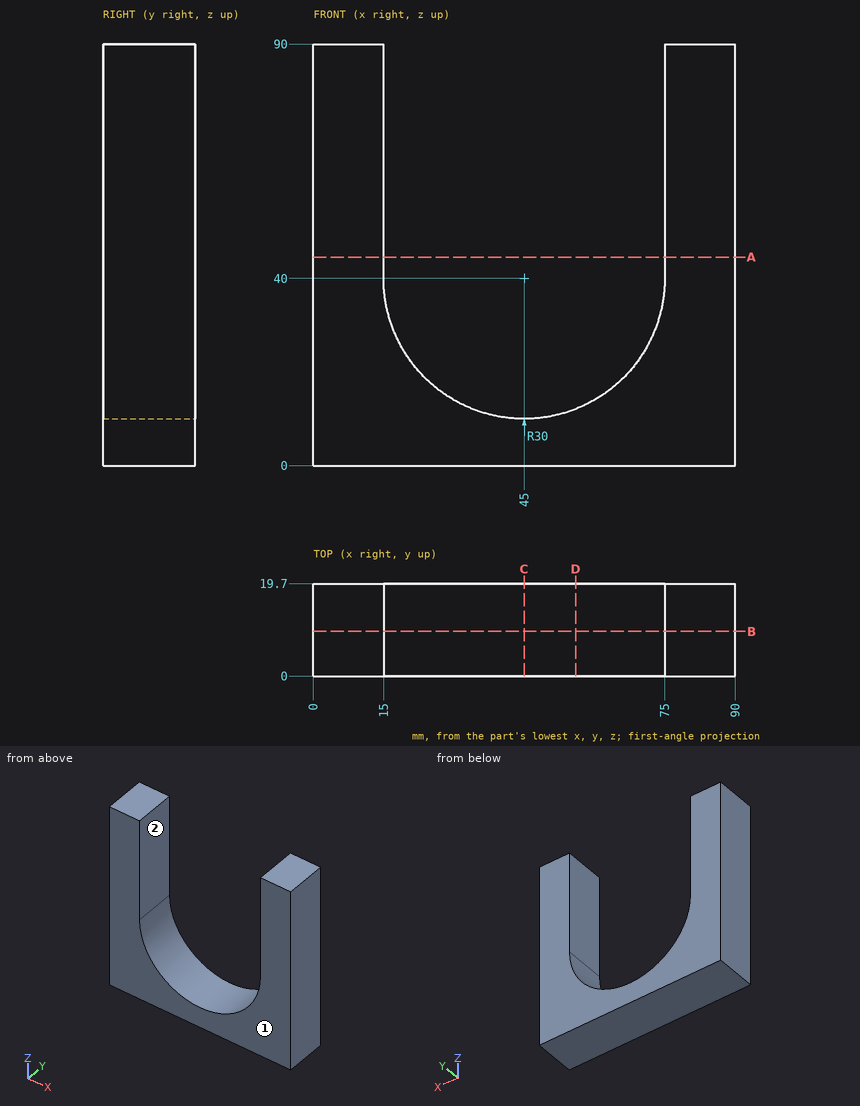
Geometry: see drawing. Coordinates: mm, zero at the bounding-box minimum. A direction names the side the tool comes from. Round coordinates to 2 decimals unless told otherwise and drop trailing zeros. Order: outer loops, then holes, each group sorted by start corner. A loop starts at its lowest first (then second) coordinate and runs counter-clockwise, first axis right, second up. Notation, with made-up numbers: (-16.5, 64.5) -> (21.5, 64.5) arc R25 ccw to (21.5, 100.5) -> close; hole circle Ø6 at (22, 1). An arc over 180 degrees is marked (long way). Use CSV: the item, a comma, the result in double quotes.
(1) Section C-C on x = 45. Return the cut outline in (y, z).
Report:
outline,"(0, 0) -> (19.7, 0) -> (19.7, 10) -> (0, 10) -> close"
(2) First-contact query: pin 1 Ø2 at (x, y) = (69, 16) entering from +Z; pin 2 Ø8 at (x, z) = (21.5, 73.5) entering from -Y; pin 3 Ø3 at (x, y) = (28, 8.5) entering from +Z. Flat tips, straight axial feed; report the tip coordinate or a pass-through.
Report:
pin 1,"z = 23.42"
pin 2,"through"
pin 3,"z = 16.38"
(3) Access query for the marked faces 1 and 2. Directions: +Z, -Z, +X, -X, +Y, -Y. A direction counts if a zero-diameter tool reaches every point of the face in a straight line with its end or side. Return the directions, or none.
Report:
face 1,"+Z, -Z, +X, -X, -Y"
face 2,"+Z, +Y, -Y"
(4) Section B-B on y = 9.5. Return the cut outline in (x, z).
Report:
outline,"(0, 0) -> (90, 0) -> (90, 90) -> (75, 90) -> (75, 40) arc R30 cw to (15, 40) -> (15, 90) -> (0, 90) -> close"
(5) Section D-D on x = 56. Return the cut outline in (y, z), and give its area (3 significant figures).
Report:
outline,"(0, 0) -> (19.7, 0) -> (19.7, 12.09) -> (0, 12.09) -> close"
area,"238 mm^2"
(6) Ray query, L1, parallel to X at y = 5, z = 71; L2, parallel to X at y = 14.75, z = 18; L3, parallel to Z at x = 43, y = 13.25. Return the intervals inside material, ascending.
Report:
L1,"0 to 15, 75 to 90"
L2,"0 to 24.6, 65.4 to 90"
L3,"0 to 10.07"
(7) Section A-A on z = 44.5. Return the cut outline in (x, y).
Report:
outline,"(0, 0) -> (15, 0) -> (15, 19.7) -> (0, 19.7) -> close; (75, 0) -> (90, 0) -> (90, 19.7) -> (75, 19.7) -> close"
